from build123d import *

# Parameters (mm, degrees)
MAIN_EXTRUSION_DEPTH = 25


with BuildPart() as part:
    # Sk Main Extrusion → Main Extrusion (new body)
    with BuildSketch(Plane.XY):
        with BuildLine():
            Line((-38.5, 4.863775977), (-25.356646534, 4.863775977))
            ThreePointArc((-25.356646534, 4.863775977), (-25.066295056, 4.956718218), (-24.883887246, 5.2009919))
            Line((-24.883887246, 5.2009919), (-23.608380992, 8.905331037))
            ThreePointArc((-23.608380992, 8.905331037), (-23.942157504, 10.351075947), (-25.387902414, 10.684852459))
            Line((-25.387902414, 10.684852459), (-28.056395253, 9.766016689))
            ThreePointArc((-28.056395253, 9.766016689), (-28.51978883, 9.839233829), (-28.718532589, 10.264198857))
            ThreePointArc((-28.718532589, 10.264198857), (-28.294243331, 12.040244762), (-27.260533906, 13.545503961))
            Line((-27.260533906, 13.545503961), (-25.833630945, 14.972406922))
            ThreePointArc((-25.833630945, 14.972406922), (-20, 17.388775977), (-14.166369055, 14.972406922))
            Line((-14.166369055, 14.972406922), (-12.739466094, 13.545503961))
            ThreePointArc((-12.739466094, 13.545503961), (-11.705756669, 12.040244762), (-11.281467411, 10.264198857))
            ThreePointArc((-11.281467411, 10.264198857), (-11.48021117, 9.839233829), (-11.943604747, 9.766016689))
            Line((-11.943604747, 9.766016689), (-14.612097586, 10.684852459))
            ThreePointArc((-14.612097586, 10.684852459), (-16.057842496, 10.351075947), (-16.391619008, 8.905331037))
            Line((-16.391619008, 8.905331037), (-15.116112754, 5.2009919))
            ThreePointArc((-15.116112754, 5.2009919), (-14.933704944, 4.956718218), (-14.643353466, 4.863775977))
            Line((-14.643353466, 4.863775977), (14.643353466, 4.863775977))
            ThreePointArc((14.643353466, 4.863775977), (14.933704944, 4.956718218), (15.116112754, 5.2009919))
            Line((15.116112754, 5.2009919), (16.391619008, 8.905331037))
            ThreePointArc((16.391619008, 8.905331037), (16.057842496, 10.351075947), (14.612097586, 10.684852459))
            Line((14.612097586, 10.684852459), (11.943604747, 9.766016689))
            ThreePointArc((11.943604747, 9.766016689), (11.48021117, 9.839233829), (11.281467411, 10.264198857))
            ThreePointArc((11.281467411, 10.264198857), (11.705756669, 12.040244762), (12.739466094, 13.545503961))
            Line((12.739466094, 13.545503961), (14.166369055, 14.972406922))
            ThreePointArc((14.166369055, 14.972406922), (20, 17.388775977), (25.833630945, 14.972406922))
            Line((25.833630945, 14.972406922), (27.260533906, 13.545503961))
            ThreePointArc((27.260533906, 13.545503961), (28.294243331, 12.040244762), (28.718532589, 10.264198857))
            ThreePointArc((28.718532589, 10.264198857), (28.51978883, 9.839233829), (28.056395253, 9.766016689))
            Line((28.056395253, 9.766016689), (25.387902414, 10.684852459))
            ThreePointArc((25.387902414, 10.684852459), (23.942157504, 10.351075947), (23.608380992, 8.905331037))
            Line((23.608380992, 8.905331037), (24.883887246, 5.2009919))
            ThreePointArc((24.883887246, 5.2009919), (25.066295056, 4.956718218), (25.356646534, 4.863775977))
            Line((25.356646534, 4.863775977), (38.5, 4.863775977))
            ThreePointArc((38.5, 4.863775977), (39.207106781, 4.570882758), (39.5, 3.863775977))
            Line((39.5, 3.863775977), (39.5, 2.277989539))
            ThreePointArc((39.5, 2.277989539), (39.423879533, 1.895306107), (39.207106781, 1.570882758))
            Line((39.207106781, 1.570882758), (32.792893219, -4.843330804))
            ThreePointArc((32.792893219, -4.843330804), (32.46846987, -5.060103556), (32.085786438, -5.136224023))
            Line((32.085786438, -5.136224023), (-32.085786438, -5.136224023))
            ThreePointArc((-32.085786438, -5.136224023), (-32.46846987, -5.060103556), (-32.792893219, -4.843330804))
            Line((-32.792893219, -4.843330804), (-39.207106781, 1.570882758))
            ThreePointArc((-39.207106781, 1.570882758), (-39.423879533, 1.895306107), (-39.5, 2.277989539))
            Line((-39.5, 2.277989539), (-39.5, 3.863775977))
            ThreePointArc((-39.5, 3.863775977), (-39.207106781, 4.570882758), (-38.5, 4.863775977))
        make_face()
    extrude(amount=-MAIN_EXTRUSION_DEPTH)


solid = part.part
Input: part model. Units: mm. Frame: model coordinates. A direction names the side the tool comes from. Give positions to 0.01 mm unless a question says otherwise; leave off trailing zeros. Order: outer loops, then holes, each group sorted by start corner. A loop starts at its lowest first (then second) coordinate and runs counter-clockwise, first axis right, second up. Notation, with made-up numbers: M -5.75,-27 L 53.25,-27 A8 cw 53.25,-13 Z; hole C 60,48.25 d9. An arc over 180 degrees is marked long. Answer as a JSON object with one key per item and string values.
1. Cut plane C-C, the plane y = 16.25. Output: boundary loops of the cut face in (x, z).
Result sheet:
{"outline": "M -24.18,-25 L -15.82,-25 L -15.82,0 L -24.18,0 Z; M 15.82,-25 L 24.18,-25 L 24.18,0 L 15.82,0 Z"}
2. First-contact query: P1, Ø10.5, axis at x = 34, z = -14.5, coming from the +Y side; P2, Ø12, axis at x = 28.5, z = -8.5, coming from the +Y side; P3, Ø4, axis at x = -30, z = -7.5, coming from the +Y side. Flat tips, straight axial feed; report the tip coordinate or a pass-through.
Result sheet:
{"P1": "y = 4.86", "P2": "y = 17", "P3": "y = 12.6"}
3. Pull-direction query (X, two-part tool) for faces 6 (the flat face through (0, 4.864, -12)), 7 (the flat face through (26.537, 14.269, -12.325)), 8 (the flat face through (-13.463, 14.269, -12.325)), 9 (the flat face through (-35.955, -1.681, -12.325)); classes: +X half, -X half, draft (parallel to the pull), parting line (faces both ways), or undercut.
Result sheet:
{"face 6": "undercut", "face 7": "+X half", "face 8": "undercut", "face 9": "-X half"}
4. Ray query, line 1 (X direction, y = 9.5, z = -11.5); line 2 (Y direction, x = -1, z = -22.25); line 3 (X direction, y = 12.75, z = -4.5). Return the intervals inside material, ascending. Write a range as [from, to].
Result sheet:
{"line 1": "[-23.54, -16.46], [16.46, 23.54]", "line 2": "[-5.14, 4.86]", "line 3": "[-27.91, -12.09], [12.09, 27.91]"}
5. Cut plane D-D, the plane y = -3.25. Output: boundary loops of the cut face in (x, z).
Result sheet:
{"outline": "M -34.39,-25 L 34.39,-25 L 34.39,0 L -34.39,0 Z"}
6. Reachability of faces 1 (the flat face through (26.74, 10.22, -12.32)), 2 (the flat face through (32, 4.864, -12)), 3 (the cylindrical face through (-11.716, 12.064, -12.325)), 4 (the flat face through (-32, 4.864, -12)), 5 (the flat face through (0, -5.136, -12)) from +Z, -Z, +X, -X, +Y, -Y: full face, straight path, thin tool, end or side. Return the list, or none.
Result sheet:
{"face 1": "+Z, -Z", "face 2": "+Z, -Z, +X", "face 3": "+Z, -Z, +Y", "face 4": "+Z, -Z, -X", "face 5": "+Z, -Z, +X, -X, -Y"}
7. Cut plane A-A, the plane y = 11.5. Output: boundary loops of the cut face in (x, z).
Result sheet:
{"outline": "M -28.5,-25 L -11.5,-25 L -11.5,0 L -28.5,0 Z; M 11.5,-25 L 28.5,-25 L 28.5,0 L 11.5,0 Z"}
8. Cut plane B-B, the plane x = 10.5. Output: boundary loops of the cut face in (y, z).
Result sheet:
{"outline": "M -5.14,-25 L 4.86,-25 L 4.86,0 L -5.14,0 Z"}
